For this review, take the finished solid that the model builds, in its own axes (mm). Face numbers are marked on the shaded views. A direction names the side the tool comes from. Coordinates: 2 decimals unless noted, no trailing zeros. Write each loop counter-clockwise with the first axis right and the second up, starting at its lowest first coordinate (ties: lowest second). Pieces come first, ordered by that corner, then holes. Notation, with made-up numbers: M 2,-38 L 49,-38 A36 ccw 49,-1 Z; hole C 88.25,12 d2. An arc over 180 degrees is marked long. One line per question, with ' | ' between items.
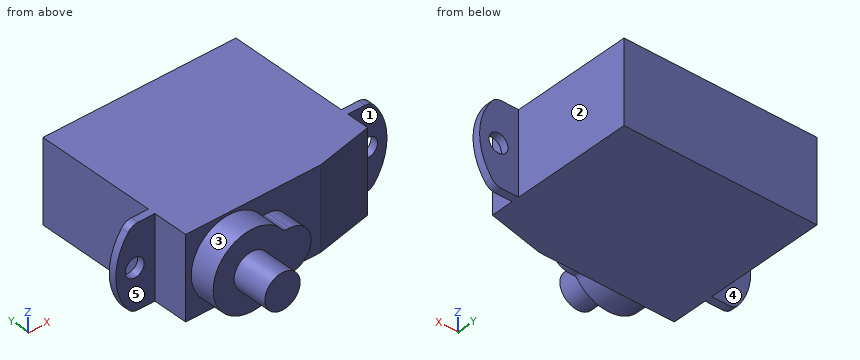
from build123d import *

# Parameters (mm, degrees)
SKETCH1_W           = 19.431
SKETCH1_H           = 8.255
BOSS_EXTRUDE1_DEPTH = 16.51
SKETCH2_R           = 0.9525
BOSS_EXTRUDE2_DEPTH = 0.762
CUT_EXTRUDE1_DEPTH  = 23.959004361
BOSS_EXTRUDE3_DEPTH = 2.54
SKETCH5_R           = 1.778
BOSS_EXTRUDE4_DEPTH = 3.556


with BuildPart() as part:
    # Sketch1 → Boss-Extrude1 (new body)
    with BuildSketch(Plane(origin=(0, 0, 0), x_dir=(1, 0, 0), z_dir=(0, 1, 0))):
        Rectangle(SKETCH1_W, SKETCH1_H)
    extrude(amount=BOSS_EXTRUDE1_DEPTH)

    # Sketch2 → Boss-Extrude2 (add)
    # profile 1 of 2: a face of its own
    with BuildSketch(Plane(origin=(0, 4.318, 0), x_dir=(1, 0, 0), z_dir=(0, 1, 0))):
        with BuildLine():
            Line((9.7155, -4.1275), (9.7155, 4.1275))
            Line((9.7155, 4.1275), (11.417923657, 4.1275))
            ThreePointArc((11.417923657, 4.1275), (11.981565763, 3.995571868), (12.428105113, 3.62719697))
            ThreePointArc((12.428105113, 3.62719697), (13.6525, 0), (12.428105113, -3.62719697))
            ThreePointArc((12.428105113, -3.62719697), (11.981565763, -3.995571868), (11.417923657, -4.1275))
            Line((11.417923657, -4.1275), (9.7155, -4.1275))
        make_face()
        with Locations(Location((11.7475, 0, 0), (0, 0, 270))):
            Circle(SKETCH2_R, mode=Mode.SUBTRACT)
    # profile 2 of 2: a face of its own
    with BuildSketch(Plane(origin=(0, 4.318, 0), x_dir=(1, 0, 0), z_dir=(0, 1, 0))):
        with BuildLine():
            Line((-9.7155, 4.1275), (-9.7155, -4.1275))
            Line((-9.7155, -4.1275), (-11.417923657, -4.1275))
            ThreePointArc((-11.417923657, -4.1275), (-11.981565763, -3.995571868), (-12.428105113, -3.62719697))
            ThreePointArc((-12.428105113, -3.62719697), (-13.6525, 0), (-12.428105113, 3.62719697))
            ThreePointArc((-12.428105113, 3.62719697), (-11.981565763, 3.995571868), (-11.417923657, 4.1275))
            Line((-11.417923657, 4.1275), (-9.7155, 4.1275))
        make_face()
        with Locations(Location((-11.7475, 0, 0), (0, 0, 270))):
            Circle(SKETCH2_R, mode=Mode.SUBTRACT)
    extrude(amount=-BOSS_EXTRUDE2_DEPTH)

    # Sketch3 → Cut-Extrude1 (cut, through all)
    with BuildSketch(Plane.XY.offset(4.1275)):
        Polygon((9.7155, 0), (3.8735, 0), (9.7155, 1.27), align=None)
    extrude(amount=-CUT_EXTRUDE1_DEPTH, mode=Mode.SUBTRACT)

    # Sketch4 → Boss-Extrude3 (add)
    with BuildSketch(Plane.XZ):
        with BuildLine():
            Line((-1.4605, 2.159), (-1.778207824, 2.159))
            ThreePointArc((-1.778207824, 2.159), (-2.003413909, 2.211647148), (-2.181941024, 2.358676301))
            ThreePointArc((-2.181941024, 2.358676301), (-9.1567, 0), (-2.181941024, -2.358676301))
            ThreePointArc((-2.181941024, -2.358676301), (-2.003413909, -2.211647148), (-1.778207824, -2.159))
            Line((-1.778207824, -2.159), (-1.4605, -2.159))
            ThreePointArc((-1.4605, -2.159), (0.6985, 0), (-1.4605, 2.159))
        make_face()
    extrude(amount=BOSS_EXTRUDE3_DEPTH)

    # Sketch5 → Boss-Extrude4 (add)
    with BuildSketch(Plane.XZ.offset(2.54)):
        with Locations(Location((-5.2705, 0, 0), (0, 0, 270))):
            Circle(SKETCH5_R)
    extrude(amount=BOSS_EXTRUDE4_DEPTH)


solid = part.part
1) We need section A-A on z = 0. State how many separate pieces and enclosed holes the cut face has, then the cut area to 3 significant figures.
Responses:
separate pieces: 3 | enclosed holes: 0 | area: 358 mm^2
2) To check wall thickness, follow line 1 along Y through (x, z) = (0.5, 1.5); line 2 along Y through (x, z) = (-3.25, 0); line 3 along X through (y, z) = (14.5, -1.5). State the ranges of each line that lie inside material, in increasing order. Write a range as [from, to].
Responses:
line 1: [0, 16.51] | line 2: [-2.54, 16.51] | line 3: [-9.72, 9.72]
3) We need section D-D on y = 8.75. State the section outline as (x, z) points.
Responses:
outline: M -9.72,-4.13 L 9.72,-4.13 L 9.72,4.13 L -9.72,4.13 Z
4) We need section C-C on z = -2.75. State the section outline as (x, y) points.
Responses:
outline: M -12.98,3.56 L -9.72,3.56 L -9.72,0 L -8.02,0 L -8.02,-2.54 L -2.52,-2.54 L -2.52,0 L 3.87,0 L 9.72,1.27 L 9.72,3.56 L 12.98,3.56 L 12.98,4.32 L 9.72,4.32 L 9.72,16.51 L -9.72,16.51 L -9.72,4.32 L -12.98,4.32 Z
5) Machinability: for the marked faces 1, 2, 3, 4 and 5, which of the approach directions +Z, -Z, +X, -X, +Y, -Y give a long, thin tool a straight path to every point of the face, cutting with its end or side? Answer none if there is none.
Responses:
face 1: +Z, -Z, +X, -Y | face 2: +Z, -Z, +X, +Y | face 3: -Y | face 4: +Z, -Z, -X, +Y | face 5: +Z, -Z, -X, -Y
6) We need section B-B on x = -0.25. State the section outline as (y, z) points, then the cut area to 3 significant figures.
Responses:
outline: M -2.54,-1.79 L 0,-1.79 L 0,-4.13 L 16.51,-4.13 L 16.51,4.13 L 0,4.13 L 0,1.79 L -2.54,1.79 Z | area: 145 mm^2
7) Insertion check: pin 1 Ø2 at (x, z) = (5.5, 2) entering from -Y; pin 2 Ø3 at (x, z) = (-12.5, 2) entering from -Y; pin 3 Ø2 at (y, z) = (-1.5, -1) entering from -X. Each pin has a flat end and moves straight along its axis. Give the tip position at first contact, or say it passes through.
Responses:
pin 1: y = 0.14 | pin 2: y = 3.56 | pin 3: x = -9.16
